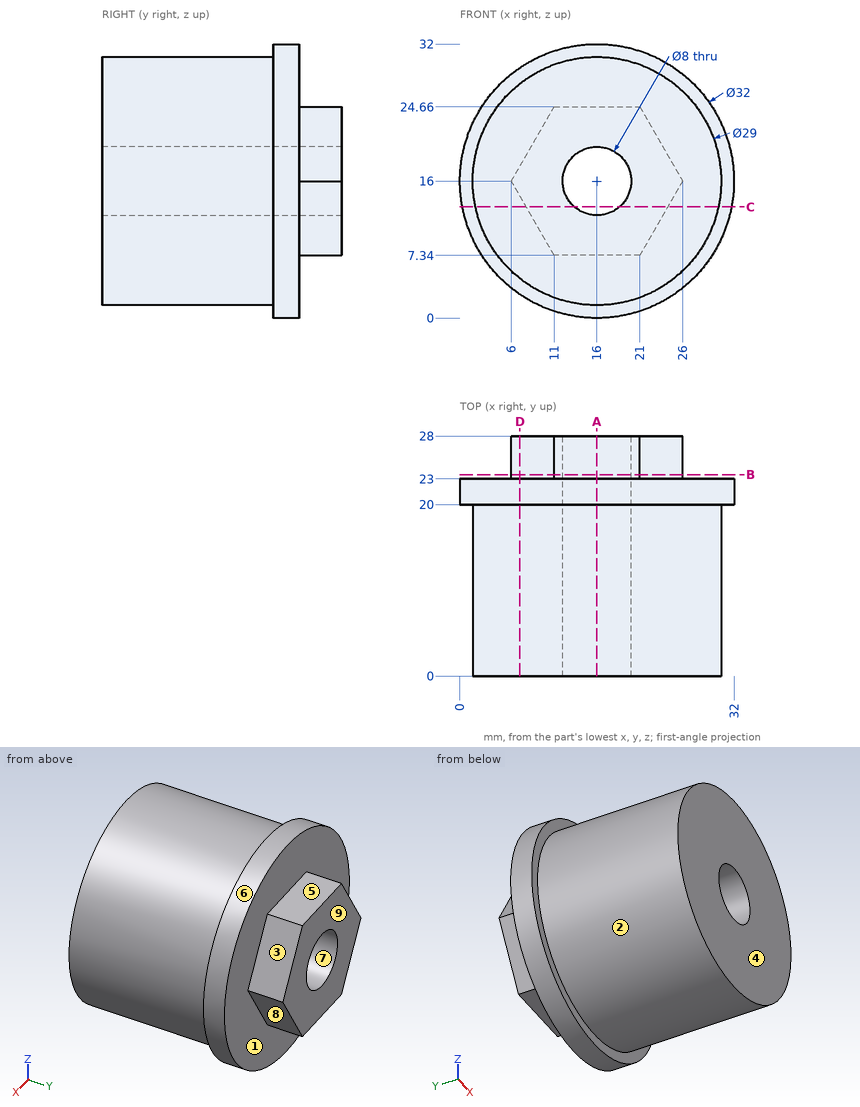
Can you work these out from the drawing? Everything is in mm from the part's minimum corner. A direction names the side the tool comes from. Coordinates: 2 decimals unless noted, no trailing zeros. Write each loop counter-clockwise with the first axis right and the second up, starting at its lowest first coordinate (ties: lowest second). Pieces come first, ordered by that corner, then holes. Notation, with made-up numbers: (27, -11) -> (43, -11) arc R15 ccw to (43, 3) -> close; hole circle Ø2 at (-33, 16.25). An arc over 180 degrees is marked (long way). Write each question's results on one line, items separated by ' | '. Start each with the question number.
Q1. If I drill on probe 1 along X at (y, z) = (14.5, 16); probe 2 along X at (y, z) = (21, 16); probe 3 along Y at (x, z) = (30, 18.5), over which ranges is the centre line in solid material (lowest first)?
Q2. Imagine slicing it at A-A (x = 16). Write out the boundary of the cut face in (y, z).
Q3. We'd pull the mould along X, two halves only. Please class the marked faces 6, 7, 8 and 9: +X half, -X half, draft (parallel to the pull), parting line (faces both ways), or undercut.
Q4. I'm going to push flat-ended pins straight in: pin 1 (4 mm diameter, centred on x = 15, y = 24.5, fed in from -Z); pin 2 (5 mm diameter, centred on y = 7, z = 23, fed in from +X); pin 3 (4 mm diameter, centred on x = 28, y = 12, fed in from -Z); pin 4 (1 mm diameter, centred on y = 9.5, z = 6.5, fed in from -X). Where does each tip first touch, or does it pass through?
Q5. On a 3-axis mill with a long thin cutter (end or side, diameter ignored), from which of +Z, -Z, +X, -X, +Y, -Y can I reach the whole of each face in a straight line? I mean the marked faces 1, 2, 3, 4 and 5. Say none if no direction works.
Q6. Imagine slicing it at D-D (x = 7). Write out the boundary of the cut face in (y, z).
Q7. Imagine slicing it at C-C (z = 13). Write out the boundary of the cut face in (x, y), then the cut area to 3 significant figures.
Q8. Imagine slicing it at B-B (y = 23.5). Write out the boundary of the cut face in (x, z).
Taken from the geometry:
1) probe 1: x = 1.5 to 12, 20 to 30.5 | probe 2: x = 0 to 12, 20 to 32 | probe 3: y = 0 to 23
2) outline: (0, 1.5) -> (20, 1.5) -> (20, 0) -> (23, 0) -> (23, 7.34) -> (28, 7.34) -> (28, 12) -> (0, 12) -> close; (0, 20) -> (28, 20) -> (28, 24.66) -> (23, 24.66) -> (23, 32) -> (20, 32) -> (20, 30.5) -> (0, 30.5) -> close
3) face 6: parting line | face 7: undercut | face 8: +X half | face 9: draft
4) pin 1: stops at z = 0 | pin 2: stops at x = 29.78 | pin 3: stops at z = 5.5 | pin 4: stops at x = 4.63
5) face 1: +Y | face 2: -Y | face 3: +Z, +X, +Y | face 4: +Z, -Z, +X, -X, -Y | face 5: +Z, +X, -X, +Y
6) outline: (0, 4.63) -> (20, 4.63) -> (20, 2.77) -> (23, 2.77) -> (23, 14.27) -> (28, 14.27) -> (28, 17.73) -> (23, 17.73) -> (23, 29.23) -> (20, 29.23) -> (20, 27.37) -> (0, 27.37) -> close
7) outline: (0.28, 20) -> (1.81, 20) -> (1.81, 0) -> (13.35, 0) -> (13.35, 28) -> (7.73, 28) -> (7.73, 23) -> (0.28, 23) -> close; (18.65, 0) -> (30.19, 0) -> (30.19, 20) -> (31.72, 20) -> (31.72, 23) -> (24.27, 23) -> (24.27, 28) -> (18.65, 28) -> close | area: 596 mm^2
8) outline: (6, 16) -> (11, 7.34) -> (21, 7.34) -> (26, 16) -> (21, 24.66) -> (11, 24.66) -> close; hole circle Ø8 at (16, 16)
